from build123d import *

# Parameters (mm, degrees)
SKETCH5_W           = 31.16
SKETCH5_H           = 43.66
BOSS_EXTRUDE2_DEPTH = 15.78
BOSS_EXTRUDE3_START = 21.83
SKETCH6_R           = 5.065
BOSS_EXTRUDE3_DEPTH = 10
SKETCH7_R           = 2.265
BOSS_EXTRUDE4_DEPTH = 10


with BuildPart() as part:
    # Sketch5 → Boss-Extrude2 (new body)
    with BuildSketch(Plane(origin=(0, 0, 0), x_dir=(1, 0, 0), z_dir=(0, 1, 0))):
        Rectangle(SKETCH5_W, SKETCH5_H)
    extrude(amount=BOSS_EXTRUDE2_DEPTH)

    # Sketch6 → Boss-Extrude3 (add)
    with BuildSketch(Plane.XY.offset(BOSS_EXTRUDE3_START)):
        with Locations((-4.139755926, 7.914788958)):
            Circle(SKETCH6_R)
        with Locations((6.643440648, 7.914788958)):
            Circle(SKETCH6_R)
    extrude(amount=BOSS_EXTRUDE3_DEPTH)

    # Sketch7 → Boss-Extrude4 (add)
    with BuildSketch(Plane(origin=(0, 0, -21.83), x_dir=(-1, 0, 0), z_dir=(0, 0, -1))):
        with Locations((-13.262092339, 7.949599191)):
            Circle(SKETCH7_R)
        with Locations((0, 7.949599191)):
            Circle(SKETCH7_R)
        with Locations((13.262092339, 7.949599191)):
            Circle(SKETCH7_R)
    extrude(amount=BOSS_EXTRUDE4_DEPTH)


solid = part.part
Could you check a few things on this model? Use its own coordinates, in mm. A direction names the side the tool comes from. Coordinates: 2 decimals unless noted, no trailing zeros. Order: outer loops, then holes, each group sorted by start corner. A loop starts at its lowest first (then second) coordinate and runs counter-clockwise, first axis right, second up. Notation, with made-up numbers: (66.5, -13) -> (79.5, -13) arc R20 cw to (79.5, 11) -> close; hole circle Ø1 at (-7, 78.5). An arc over 180 degrees is marked (long way). One line per item, written item: value. Start each with the question number.
1) Imagine slicing it at B-B on z = -27. List the corners of the cut face in (x, y) for me (3 decimals), plus the area to 3 significant figures.
2) I'm going to push flat-ended pins straight in: pin 1 (5 mm diameter, centred on x = 11.5, y = 3, fed in from +Z); pin 2 (2 mm diameter, centred on y = 4.5, z = 23.5, fed in from -X); pin 3 (4.5 mm diameter, centred on x = -4, y = 5.5, fed in from -Z). Where does each tip first touch, or does it pass through?
3) Which directions (+Z, -Z, +X, -X, +Y, -Y) give clear straight access to the entire face, cutting with the end or side of a thin tool? Please do faces 1 (the flat face through (13, 8, -31.83)), 2 (the cylindrical face through (-5.24, 2.97, 26.76)), 3 (the cylindrical face through (12.044, 9.859, -26.76)).
4) Imagine slicing it at C-C on y = 9.5. List the corners of the cut face in (x, z) for me, plus the area to 3 significant figures.
5) We'd pull the mould along X, two halves only. Please class faces 4 (the flat face through (7, 8, 31.83)), 5 (the flat face through (-15.58, 8, 0)), 6 (the flat face through (-4, 8, -21.83)): +X half, -X half, draft (parallel to the pull), parting line (faces both ways), or undercut.
6) Imagine slicing it at D-D on x = -3. List the corners of the cut face in (y, z) for me, plus the area to 3 significant figures.
7) Imagine slicing it at A-A on x = 3. List the corners of the cut face in (y, z) for me.
8) If I drill on L1, parallel to Z at x = 14, y = 14.25; L2, parallel to Z at x = 10, y = 8.5; L3, parallel to Y at x = 0, z = -28, over which ranges is the centre line in solid material (lowest first)? Write a range as [from, to].
Answer list:
1. outline: circle Ø4.53 at (-13.262, 7.95); circle Ø4.53 at (0, 7.95); circle Ø4.53 at (13.262, 7.95)
1. area: 48.4 mm2
2. pin 1: stops at z = 31.83
2. pin 2: stops at x = -8.59
2. pin 3: stops at z = -21.83
3. face 1: -Z, +X, -X, +Y, -Y
3. face 2: +Z
3. face 3: -Z
4. outline: (-15.58, -21.83) -> (-14.91, -21.83) -> (-14.91, -31.83) -> (-11.61, -31.83) -> (-11.61, -21.83) -> (-1.65, -21.83) -> (-1.65, -31.83) -> (1.65, -31.83) -> (1.65, -21.83) -> (11.61, -21.83) -> (11.61, -31.83) -> (14.91, -31.83) -> (14.91, -21.83) -> (15.58, -21.83) -> (15.58, 21.83) -> (11.45, 21.83) -> (11.45, 31.83) -> (1.83, 31.83) -> (1.83, 21.83) -> (0.67, 21.83) -> (0.67, 31.83) -> (-8.95, 31.83) -> (-8.95, 21.83) -> (-15.58, 21.83) -> close
4. area: 1,650 mm2
5. face 4: draft
5. face 5: -X half
5. face 6: undercut
6. outline: (0, -21.83) -> (15.78, -21.83) -> (15.78, 21.83) -> (12.85, 21.83) -> (12.85, 31.83) -> (2.98, 31.83) -> (2.98, 21.83) -> (0, 21.83) -> close
6. area: 788 mm2
7. outline: (0, -21.83) -> (15.78, -21.83) -> (15.78, 21.83) -> (11.43, 21.83) -> (11.43, 31.83) -> (4.4, 31.83) -> (4.4, 21.83) -> (0, 21.83) -> close
8. L1: z = [-21.83, 21.83]
8. L2: z = [-21.83, 31.83]
8. L3: y = [5.68, 10.21]
